Verification items for the finished model (mm, model axes). A direction names the side the tool comes from. Coordinates: 2 decimals unless noted, no trailing zeros. Write each loop counter-clockwise with the first axis right and the second up, starting at its lowest first coordinate (ties: lowest second). Pieces come first, ordered by that corner, then holes. Notation, with made-up numbers: M -26,-27.75 L -6,-27.75 A22 ccw -6,-9.75 Z; hole C -7.75,-37.75 d10. An arc over 180 degrees is marked long. One line per item, written item: value.
```python
from build123d import *

# Parameters (mm, degrees)
SKETCH2_W           = 61
SKETCH2_H           = 61
BOSS_EXTRUDE1_DEPTH = 12
SKETCH4_R           = 10
CUT_EXTRUDE3_DEPTH  = 10
CUT_EXTRUDE5_DEPTH  = 10
FILLET2_SIZE        = 2
FILLET3_R           = 5


with BuildPart() as part:
    # Sketch2 → Boss-Extrude1 (new body)
    with BuildSketch(Plane(origin=(0, 0, 0), x_dir=(1, 0, 0), z_dir=(0, 1, 0))):
        Rectangle(SKETCH2_W, SKETCH2_H)
    extrude(amount=BOSS_EXTRUDE1_DEPTH)

    # Sketch4 → Cut-Extrude3 (cut)
    with BuildSketch(Plane(origin=(0, 12, 0), x_dir=(1, 0, 0), z_dir=(0, 1, 0))):
        with Locations((30.5, -30.5)):
            Circle(SKETCH4_R)
        with Locations((-30.5, -30.5)):
            Circle(SKETCH4_R)
        with Locations((-30.5, 30.5)):
            Circle(SKETCH4_R)
        with Locations((30.5, 30.5)):
            Circle(SKETCH4_R)
    extrude(amount=-CUT_EXTRUDE3_DEPTH, mode=Mode.SUBTRACT)

    # Sketch8 → Cut-Extrude5 (cut)
    with BuildSketch(Plane.XZ):
        with BuildLine():
            Line((-18.667840434, -28.5), (18.667840434, -28.5))
            ThreePointArc((18.667840434, -28.5), (22.014718626, -22.014718626), (28.5, -18.667840434))
            Line((28.5, -18.667840434), (28.5, 18.667840434))
            ThreePointArc((28.5, 18.667840434), (22.014718626, 22.014718626), (18.667840434, 28.5))
            Line((18.667840434, 28.5), (-18.667840434, 28.5))
            ThreePointArc((-18.667840434, 28.5), (-22.014718626, 22.014718626), (-28.5, 18.667840434))
            Line((-28.5, 18.667840434), (-28.5, -18.667840434))
            ThreePointArc((-28.5, -18.667840434), (-22.014718626, -22.014718626), (-18.667840434, -28.5))
        make_face()
    extrude(amount=-CUT_EXTRUDE5_DEPTH, mode=Mode.SUBTRACT)

    # Fillet2
    fillet2_edges = [part.edges().sort_by_distance(p)[0] for p in [
        (30.5, 12, 0),
        (0, 12, -30.5),
        (-30.5, 12, 0),
        (0, 12, 30.5),
        (23.428932188, 12, -23.428932188),
        (-23.428932188, 12, -23.428932188),
        (-23.428932188, 12, 23.428932188),
        (23.428932188, 12, 23.428932188),
    ]]
    chamfer(fillet2_edges, length=FILLET2_SIZE)

    # Sketch15 → M3x0.5 Tapped Hole1 (revolve, cut)
    with BuildSketch(Plane(origin=(26.5, 2, 26.5), x_dir=(0, 0, 1), z_dir=(1, 0, 0))):
        Polygon((0, 0), (0, 8.251075774), (1.25, 7.5), (1.25, 0), align=None)
    m3x0_5_tapped_hole1 = revolve(axis=Axis((26.5, 8.35, 26.5), (0, -1, 0)), mode=Mode.SUBTRACT)

    # Mirror1: M3x0.5 Tapped Hole1 across plane
    add(m3x0_5_tapped_hole1.mirror(Plane.XY), mode=Mode.SUBTRACT)

    # Mirror2: M3x0.5 Tapped Hole1 across plane
    add(m3x0_5_tapped_hole1.mirror(Plane(origin=(0, 0, 0), x_dir=(0, 0, 1), z_dir=(1, 0, 0))), mode=Mode.SUBTRACT)

    # Mirror2 copy 1 sketch → Mirror2 copy 1 (revolve, cut)
    with BuildSketch(Plane(origin=(-26.5, 2, -26.5), x_dir=(0, 0, -1), z_dir=(-1, 0, 0))):
        Polygon((0, 0), (0, 8.251075774), (1.25, 7.5), (1.25, 0), align=None)
    revolve(axis=Axis((-26.5, 8.35, -26.5), (0, -1, 0)), mode=Mode.SUBTRACT)

    # Fillet3
    fillet3_edges = [part.edges().sort_by_distance(p)[0] for p in [
        (28.5, 5, -18.667840434),
        (18.667840434, 5, -28.5),
        (-18.667840434, 5, -28.5),
        (-28.5, 5, -18.667840434),
        (-28.5, 5, 18.667840434),
        (-18.667840434, 5, 28.5),
        (18.667840434, 5, 28.5),
        (28.5, 5, 18.667840434),
    ]]
    fillet(fillet3_edges, radius=FILLET3_R)


solid = part.part
```
Item 1: Cross-section at D-D, the plane y = 11.25. Enter the section's corners in (x, z), and give its area (3 significant figures).
The answers:
outline: M -29.25,-19.32 A11.25 cw -19.32,-29.25 L 19.32,-29.25 A11.25 cw 29.25,-19.32 L 29.25,19.32 A11.25 cw 19.32,29.25 L -19.32,29.25 A11.25 cw -29.25,19.32 Z
area: 3,130 mm²
Item 2: Access from +Z, -Z, +X, -X, +Y, -Y to the whole of each face (thin tool, end or side, straight path). Record for faces 1 (the face through (-23.51, 6.06, -23.35)), 2 (the face through (22.964, 10.542, -23.128)), 3 (the face through (-21.97, 4.93, 22.06)).
The answers:
face 1: -Z, -X, +Y
face 2: -Z, +X, +Y
face 3: -Y
Item 3: Go/stop test with flat-tipped pins: P1, Ø5, axis at x = 25, z = 24.5, coming from the +Y side; P2, Ø2, axis at x = 26.5, z = -26.5, coming from the -Y side; P3, Ø4, axis at x = 26.5, z = 26.5, coming from the +Y side. Record where each tip stops, or that it passes through.
The answers:
P1: stops at y = 10.64
P2: passes through
P3: stops at y = 2
Item 4: Scan lines: line 1 (Z direction, x = -15, y = 9); line 2 (X direction, y = 1.1, z = 26.5). Record each from-to range of solid material in increasing order.
The answers:
line 1: z = -30.5 to -28.5, 28.5 to 30.5
line 2: x = -30.5 to -27.75, -25.25 to -19.01, 19.01 to 25.25, 27.75 to 30.5
Item 5: Cross-section at B-B, the plane z = 6. Enter the section's corners in (x, y), and give its area (3 significant figures).
The answers:
outline: M -30.5,0 L -28.5,0 L -28.5,10 L 28.5,10 L 28.5,0 L 30.5,0 L 30.5,10 L 28.5,12 L -28.5,12 L -30.5,10 Z
area: 158 mm²
Item 6: Cross-section at A-A, the plane y = 6.5. Enter the section's corners in (x, z), and give its area (3 significant figures).
The answers:
outline: M -30.5,-20.5 A10 cw -20.5,-30.5 L 20.5,-30.5 A10 cw 30.5,-20.5 L 30.5,20.5 A10 cw 20.5,30.5 L -20.5,30.5 A10 cw -30.5,20.5 Z; hole M -28.5,-15.01 A5 ccw -25.56,-19.56 A12 cw -19.56,-25.56 A5 ccw -15.01,-28.5 L 15.01,-28.5 A5 ccw 19.56,-25.56 A12 cw 25.56,-19.56 A5 ccw 28.5,-15.01 L 28.5,15.01 A5 ccw 25.56,19.56 A12 cw 19.56,25.56 A5 ccw 15.01,28.5 L -15.01,28.5 A5 ccw -19.56,25.56 A12 cw -25.56,19.56 A5 ccw -28.5,15.01 Z
area: 453 mm²
Item 7: Cross-section at C-C, the plane x = -7.5. Enter the section's corners in (y, z), and give its area (3 significant figures).
The answers:
outline: M 0,-30.5 L 10,-30.5 L 12,-28.5 L 12,28.5 L 10,30.5 L 0,30.5 L 0,28.5 L 10,28.5 L 10,-28.5 L 0,-28.5 Z
area: 158 mm²
Item 8: Draft check along X on faces 4 (the face through (-29.5, 11, 0.3)), 5 (the face through (22.06, 4.93, 21.97)), 6 (the face through (-22.06, 4.93, -21.97)), 7 (the face through (29.5, 11, 0.3)). Enter one of: released by +X, released by -X, zero draft, split by the parting line, or undercut.
The answers:
face 4: released by -X
face 5: undercut
face 6: undercut
face 7: released by +X
